```python
from build123d import *

# Parameters (mm, degrees)
F0_W     = 68
F0_H     = 70
F0_R     = 1.6
F0_R_2   = 0.95
F1_DEPTH = 3


with BuildPart() as f1:
    # F0 (on Front) → F1 (new body)
    with BuildSketch(Plane.XZ):
        with Locations((3.531757, -8.419635)):
            Rectangle(F0_W, F0_H)
        with Locations((-26.468243, -28.419635)):
            Circle(F0_R, mode=Mode.SUBTRACT)
        with Locations((-16.468243, -26.419635)):
            Circle(F0_R_2, mode=Mode.SUBTRACT)
        with Locations((28.531757, -26.419635)):
            Circle(F0_R_2, mode=Mode.SUBTRACT)
        with Locations((-26.468243, -8.419635)):
            Circle(F0_R, mode=Mode.SUBTRACT)
        with Locations((-26.468243, 11.580365)):
            Circle(F0_R, mode=Mode.SUBTRACT)
        with Locations((-16.468243, 12.580365)):
            Circle(F0_R_2, mode=Mode.SUBTRACT)
        Polygon((-17.518243, 15.556515), (-17.518243, 23.106515), (29.481757, 23.106515), (29.481757, 15.530365), (25.581757, 15.530365), (25.581757, 9.630365), (29.481757, 9.630365), (29.481757, -23.469635), (25.581757, -23.469635), (25.581757, -29.369635), (29.481757, -29.369635), (29.481757, -37.893485), (-17.518243, -37.893485), (-17.518243, -29.343485), (-13.518243, -29.343485), (-13.518243, -23.469635), (-17.518243, -23.469635), (-17.518243, 9.630365), (-13.518243, 9.630365), (-13.518243, 15.556515), align=None, mode=Mode.SUBTRACT)
        with Locations((28.531757, 12.580365)):
            Circle(F0_R_2, mode=Mode.SUBTRACT)
    extrude(amount=F1_DEPTH)


solid = f1.part
```
Part model, mm, in its own coordinate system. A direction names the side the tool comes from. Round coordinates to 2 decimals unless told otherwise and drop trailing zeros. Loops run counter-clockwise (first coordinate to the right, second up) from the corner with the lowest first, then second, coordinate; pieces in that order, holes last. Notation, with made-up numbers: (-31.75, -29.75) -> (24.25, -29.75) arc R8 ccw to (24.25, -18.75) -> close; hole circle Ø3 at (-40, -36.75). An arc over 180 degrees is marked (long way). Use CSV: the item, a comma, the result in double quotes. Start each with the question number.
1) Cut at C-C, the plane y = -1.6. Give the number of separate pieces and of enclosed holes in the cut face, plus the area to 3 significant figures.
2) Drop flat-ended pins along their axis: P1, Ø5, axis at x = -26.47, z = -8.42, coming from the -Y side; P2, Ø1.1, axis at x = -16.47, z = -26.42, coming from the +Y side. Give the stop position or say it passes through.
3) Which spindle directions (+Z, -Z, +X, -X, +Y, -Y) get a long thin tool onto all of the face, cutting with end or side? Do faces 4 (the flat face through (-20, -3, -8)), 5 (the flat face through (29.482, -1, -34)). Say none if no direction does.
4) Pull direction X, two halves, no side cores. Call faces 1 (the flat face through (-30.468, -1, -9)), 2 (the flat face through (3, -1, 26.58)), 3 (the flat face through (6, -1, -37.893)): +X half, -X half, draft (parallel to the pull), parting line (faces both ways), or undercut.
5) Wall check: L1, parallel to X at y = -2.7, z = -31.5; L2, parallel to X at y = -1, z = 14; L3, parallel to Z at x = 15, y = -0.3. Give the ranges that are in metal, low to high. Write a range as [from, to].
6) Cut at B-B, the plane z = -17. Write the cut outline in (x, y), plus the area to 3 significant figures.
7) Cut at A-A, the plane x = 5. Write the cut outline in (y, z), plus the area to 3 significant figures.
Determined:
1,separate pieces,"1"
1,enclosed holes,"8"
1,area,"1,950 mm2"
2,P1,"stops at y = -3"
2,P2,"passes through"
3,face 4,"+Z, -Z, +X, -X, -Y"
3,face 5,"+Y, -Y"
4,face 1,"-X half"
4,face 2,"draft"
4,face 3,"undercut"
5,L1,"x = [-30.47, -17.52], [29.48, 37.53]"
5,L2,"x = [-30.47, -13.52], [25.58, 37.53]"
5,L3,"z = [-43.42, -37.89], [23.11, 26.58]"
6,outline,"(-30.47, -3) -> (-17.52, -3) -> (-17.52, 0) -> (-30.47, 0) -> close; (29.48, -3) -> (37.53, -3) -> (37.53, 0) -> (29.48, 0) -> close"
6,area,"63.0 mm2"
7,outline,"(-3, -43.42) -> (0, -43.42) -> (0, -37.89) -> (-3, -37.89) -> close; (-3, 23.11) -> (0, 23.11) -> (0, 26.58) -> (-3, 26.58) -> close"
7,area,"27.0 mm2"
